from build123d import *

# Parameters (mm, degrees)
SKETCH1_R           = 5.207
BOSS_EXTRUDE1_DEPTH = 3.175
SKETCH2_W           = 10.16
SKETCH2_H           = 3.175
BOSS_EXTRUDE2_DEPTH = 12.7
FILLET1_R           = 2.54
CUT_EXTRUDE1_DEPTH  = 51.596342012
FILLET2_R           = 1.27


with BuildPart() as part:
    # Sketch1 → Boss-Extrude1 (new body)
    with BuildSketch(Plane.XY):
        with BuildLine():
            Line((-40, 8.89), (40, 8.89))
            ThreePointArc((40, 8.89), (48.89, 0), (40, -8.89))
            Line((40, -8.89), (-40, -8.89))
            ThreePointArc((-40, -8.89), (-48.89, 0), (-40, 8.89))
        make_face()
        with Locations((-40, 0)):
            Circle(SKETCH1_R, mode=Mode.SUBTRACT)
        with Locations((40, 0)):
            Circle(SKETCH1_R, mode=Mode.SUBTRACT)
    extrude(amount=BOSS_EXTRUDE1_DEPTH)

    # Sketch2 → Boss-Extrude2 (add)
    with BuildSketch(Plane.XY):
        with Locations((24.13, -7.3025)):
            Rectangle(SKETCH2_W, SKETCH2_H)
        with Locations((-24.13, -7.3025)):
            Rectangle(SKETCH2_W, SKETCH2_H)
    extrude(amount=BOSS_EXTRUDE2_DEPTH)

    # Fillet1
    fillet1_edges = [part.edges().sort_by_distance(p)[0] for p in [
        (-24.13, -5.715, 3.175),
        (24.13, -5.715, 3.175),
    ]]
    fillet(fillet1_edges, radius=FILLET1_R)

    # Sketch3 → Cut-Extrude1 (cut, through all)
    with BuildSketch(Plane.XY.offset(3.175)):
        with BuildLine():
            Line((-31.75, -0.635), (-32.27906845, -0.635))
            ThreePointArc((-32.27906845, -0.635), (-32.98887591, 3.295473864), (-35.562263077, 6.35))
            Line((-35.562263077, 6.35), (-3.619187949, 6.35))
            Line((-3.619187949, 6.35), (-16.51, -6.35))
            Line((-16.51, -6.35), (-16.51, -0.635))
            Line((-16.51, -0.635), (-31.75, -0.635))
        make_face()
        with BuildLine():
            Line((31.75, -0.635), (32.27906845, -0.635))
            ThreePointArc((32.27906845, -0.635), (32.98887591, 3.295473864), (35.562263077, 6.35))
            Line((35.562263077, 6.35), (3.997987617, 6.35))
            Line((3.997987617, 6.35), (16.51, -6.35))
            Line((16.51, -6.35), (16.51, -0.635))
            Line((16.51, -0.635), (31.75, -0.635))
        make_face()
        Polygon((-12.890812051, -6.35), (0, 6.35), (12.512012383, -6.35), align=None)
    extrude(amount=-CUT_EXTRUDE1_DEPTH, mode=Mode.SUBTRACT)

    # Fillet2
    fillet2_edges = [part.edges().sort_by_distance(p)[0] for p in [
        (35.562263077, 6.35, 1.5875),
        (32.27906845, -0.635, 1.5875),
        (16.51, -0.635, 1.5875),
        (16.51, -6.35, 1.5875),
        (3.997987617, 6.35, 1.5875),
        (12.512012383, -6.35, 1.5875),
        (-12.890812051, -6.35, 1.5875),
        (0, 6.35, 1.5875),
        (-32.27906845, -0.635, 1.5875),
        (-35.562263077, 6.35, 1.5875),
        (-3.619187949, 6.35, 1.5875),
        (-16.51, -6.35, 1.5875),
        (-16.51, -0.635, 1.5875),
    ]]
    fillet(fillet2_edges, radius=FILLET2_R)


solid = part.part
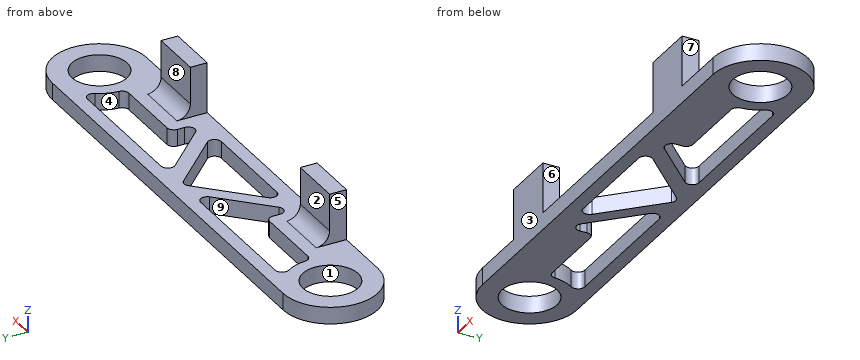
Model file for the job. Use its own axes, mm. Face numbers are marked on the shaded views. A direction names the side the tool comes from. Coordinates: 2 decimals unless noted, no trailing zeros. Write each loop counter-clockwise with the first axis right and the second up, starting at its lowest first coordinate (ties: lowest second). Pieces come first, ordered by that corner, then holes. Notation, with made-up numbers: (30.5, 33.5) -> (75.5, 33.5) arc R27 ccw to (75.5, 71.5) -> close; hole circle Ø6 at (26, 60). An arc over 180 degrees is marked (long way). One line per item, written item: value. Start each with the question number.
1) Which spindle directions (+Z, -Z, +X, -X, +Y, -Y) get a long thin tool onto all of the face, cutting with end or side? Do the marked faces 5, 6, 7, 8 and 9. Say none if no direction does.
2) Flat gauge pins, fed straight in: pin 1 Ø1.7 at (y, z) = (-7, 5.5) entering from +X; pin 2 Ø1.5 at (y, z) = (3.5, 1.5) entering from +X; pin 3 Ø3 at (x, z) = (25, 5) entering from +Y. Where does each tip first touch, or does it go through?
3) Pull direction Y, two halves, no side cores. Call the marked faces 1, 2, 3 and 4: +Y half, -Y half, draft (parallel to the pull), parting line (faces both ways), or undercut.
4) Slice it at D-D on x = 8. Write the cut outline in (y, z) (3 decimals), then the cut area to 3 significant figures.
5) Slice it at C-C on x = -20.5. Write the cut outline in (y, z) (3 decimals), then the cut area to 3 significant figures.
6) Probe probe 1 along X at (y, z) = (-7.25, 5.75); probe 2 along X at (y, z) = (-4.75, 1.75); probe 3 along Y at (x, z) = (-40, 0.85). List the from-to ranges inside material, lowest first.
7) Slice it at B-B on z = 1.25. Count the separate pieces of the cut face and the enclosed holes in it, then the cut area to 3 significant figures.
8) Slice it at A-A on z = 7. Write the cut outline in (x, y) (3 decimals), then the cut area to 3 significant figures.
Answers follow:
1. face 5: +Z, -X, +Y, -Y
1. face 6: +Z, +Y, -Y
1. face 7: +Z, +X, +Y, -Y
1. face 8: +Z, +X, -X, +Y
1. face 9: +Z, -Z
2. pin 1: x = 29.21
2. pin 2: x = 48.45
2. pin 3: y = -4.42
3. face 1: undercut
3. face 2: +Y half
3. face 3: -Y half
3. face 4: undercut
4. outline: (-8.89, 0) -> (-6.35, 0) -> (-6.35, 3.175) -> (-8.89, 3.175) -> close; (-1.77, 0) -> (2.288, 0) -> (2.288, 3.175) -> (-1.77, 3.175) -> close; (6.35, 0) -> (8.89, 0) -> (8.89, 3.175) -> (6.35, 3.175) -> close
4. area: 29.0 mm2
5. outline: (-8.89, 0) -> (-0.635, 0) -> (-0.635, 3.175) -> (-3.175, 3.175) arc R2.54 cw to (-5.715, 5.715) -> (-5.715, 12.7) -> (-8.89, 12.7) -> close; (6.35, 0) -> (8.89, 0) -> (8.89, 3.175) -> (6.35, 3.175) -> close
5. area: 65.9 mm2
6. probe 1: -29.21 to -19.05, 19.05 to 29.21
6. probe 2: -47.51 to -42.13, -37.87 to -11.02, 10.7 to 37.87, 42.13 to 47.51
6. probe 3: -8.89 to -5.21, 5.21 to 8.89
7. separate pieces: 1
7. enclosed holes: 5
7. area: 961 mm2
8. outline: (-29.21, -8.89) -> (-19.05, -8.89) -> (-19.05, -5.715) -> (-29.21, -5.715) -> close; (19.05, -8.89) -> (29.21, -8.89) -> (29.21, -5.715) -> (19.05, -5.715) -> close
8. area: 64.5 mm2
